from build123d import *

# Parameters (mm, degrees)
AUFSATZ_LINEAR_AUSTRAGEN1_DEPTH      = 10
SCHNITT_LINEAR_START                 = -0.7
SCHNITT_LINEAR_AUSTRAGEN1_DEPTH      = 0.7
SKIZZE5_W                            = 196
SKIZZE5_H                            = 8.65
AUFSATZ_LINEAR_AUSTRAGEN2_DEPTH      = 10
SCHNITT_LINEAR_AUSTRAGEN2_DEPTH      = 0.7
SCHNITT_LINEAR_AUSTRAGEN3_DEPTH      = 10
SCHNITT_LINEAR_AUSTRAGEN3_DEPTH_BACK = 10
BOHRUNG1_D                           = 6
BOHRUNG2_D                           = 4.134
BOHRUNG2_DEPTH                       = 10
BOHRUNG2_CSINK_D                     = 5
BOHRUNG2_CSINK_ANGLE                 = 90
BOHRUNG3_D                           = 4.134
BOHRUNG3_DEPTH                       = 10
BOHRUNG3_CSINK_D                     = 5
BOHRUNG3_CSINK_ANGLE                 = 90


with BuildPart() as part:
    # Skizze1 → Rotation1 (revolve)
    with BuildSketch(Plane.XY, mode=Mode.PRIVATE) as rotation1_sk:
        with BuildLine():
            Line((0, 0), (0, 6.8))
            Line((0, 6.8), (0.2, 7))
            Line((0.2, 7), (1, 7))
            Line((1, 7), (2, 8))
            Line((2, 8), (11.95, 8))
            Line((11.95, 8), (12.865685425, 7.084314575))
            ThreePointArc((12.865685425, 7.084314575), (13.125224104, 6.910896374), (13.43137085, 6.85))
            Line((13.43137085, 6.85), (14.2, 6.85))
            ThreePointArc((14.2, 6.85), (14.765685425, 7.084314575), (15, 7.65))
            Line((15, 7.65), (15, 8))
            Line((15, 8), (17, 8))
            Line((17, 8), (17, 0))
            Line((17, 0), (0, 0))
        make_face()
    revolve(rotation1_sk.sketch.rotate(Axis((17, 0, 0), (-1, 0, 0)), 270), axis=Axis((17, 0, 0), (-1, 0, 0)))

    # Skizze2 → Aufsatz-Linear austragen1 (add)
    with BuildSketch(Plane(origin=(17, 0, 0), x_dir=(0, 0, -1), z_dir=(1, 0, 0))):
        with BuildLine():
            Line((4.75, 8.977054082), (4.75, 9.6))
            ThreePointArc((4.75, 9.6), (4.632842712, 9.882842712), (4.35, 10))
            Line((4.35, 10), (-4.35, 10))
            ThreePointArc((-4.35, 10), (-4.632842712, 9.882842712), (-4.75, 9.6))
            Line((-4.75, 9.6), (-4.75, 8.977054082))
            ThreePointArc((-4.75, 8.977054082), (-4.791034545, 8.825604773), (-4.902912621, 8.715586488))
            ThreePointArc((-4.902912621, 8.715586488), (0, -10), (4.902912621, 8.715586488))
            ThreePointArc((4.902912621, 8.715586488), (4.791034545, 8.825604773), (4.75, 8.977054082))
        make_face()
    extrude(amount=AUFSATZ_LINEAR_AUSTRAGEN1_DEPTH)

    # Skizze3 → Schnitt-Rotation1 (revolve, cut)
    with BuildSketch(Plane(origin=(23, 0, 0), x_dir=(0, 0, -1), z_dir=(1, 0, 0)), mode=Mode.PRIVATE) as schnitt_rotation1_sk:
        Polygon((6.5, 9.5), (8.25, 9.5), (8.25, 5.4), (8, 5.4), (8, 5.3), (7.8, 5.5), (6.5, 5.5), align=None)
    revolve(schnitt_rotation1_sk.sketch.rotate(Axis((23, 5.5, -6.5), (0, 1, 0)), 180), axis=Axis((23, 5.5, -6.5), (0, 1, 0)), mode=Mode.SUBTRACT)

    # Skizze4 → Schnitt-Linear austragen1 (cut)
    with BuildSketch(Plane(origin=(0, 5.5, 0), x_dir=(1, 0, 0), z_dir=(0, 1, 0)).offset(SCHNITT_LINEAR_START)):
        with BuildLine():
            Line((23.3, 5.030306154), (23.3, 7.969693846))
            ThreePointArc((23.3, 7.969693846), (23, 8), (22.7, 7.969693846))
            Line((22.7, 7.969693846), (22.7, 5.030306154))
            ThreePointArc((22.7, 5.030306154), (23, 5), (23.3, 5.030306154))
        make_face()
    extrude(amount=SCHNITT_LINEAR_AUSTRAGEN1_DEPTH, mode=Mode.SUBTRACT)

    # Skizze5 → Rotation2 (revolve)
    with BuildSketch(Plane.XY, mode=Mode.PRIVATE) as rotation2_sk:
        with Locations((125, 4.325)):
            Rectangle(SKIZZE5_W, SKIZZE5_H)
    revolve(rotation2_sk.sketch.rotate(Axis((223, 0, 0), (-1, 0, 0)), 270), axis=Axis((223, 0, 0), (-1, 0, 0)))

    # Skizze6 → Aufsatz-Linear austragen2 (add)
    with BuildSketch(Plane(origin=(223, 0, 0), x_dir=(0, 0, -1), z_dir=(1, 0, 0))):
        with BuildLine():
            Line((4.75, 8.977054082), (4.75, 9.6))
            ThreePointArc((4.75, 9.6), (4.632842712, 9.882842712), (4.35, 10))
            Line((4.35, 10), (-4.35, 10))
            ThreePointArc((-4.35, 10), (-4.632842712, 9.882842712), (-4.75, 9.6))
            Line((-4.75, 9.6), (-4.75, 8.977054082))
            ThreePointArc((-4.75, 8.977054082), (-4.791034545, 8.825604773), (-4.902912621, 8.715586488))
            ThreePointArc((-4.902912621, 8.715586488), (0, -10), (4.902912621, 8.715586488))
            ThreePointArc((4.902912621, 8.715586488), (4.791034545, 8.825604773), (4.75, 8.977054082))
        make_face()
    extrude(amount=AUFSATZ_LINEAR_AUSTRAGEN2_DEPTH)

    # Skizze7 → Schnitt-Rotation2 (revolve, cut)
    with BuildSketch(Plane(origin=(225.35, 0, 0), x_dir=(0, 0, -1), z_dir=(1, 0, 0)), mode=Mode.PRIVATE) as schnitt_rotation2_sk:
        Polygon((6.5, 9.5), (8.25, 9.5), (8.25, 5.4), (8, 5.4), (8, 5.3), (7.8, 5.5), (6.5, 5.5), align=None)
    revolve(schnitt_rotation2_sk.sketch.rotate(Axis((225.35, 5.5, -6.5), (0, 1, 0)), 180), axis=Axis((225.35, 5.5, -6.5), (0, 1, 0)), mode=Mode.SUBTRACT)

    # Skizze8 → Schnitt-Linear austragen2 (cut)
    with BuildSketch(Plane(origin=(0, 5.5, 0), x_dir=(1, 0, 0), z_dir=(0, 1, 0)).offset(SCHNITT_LINEAR_START)):
        with BuildLine():
            Line((225.65, 5.030306154), (225.65, 7.969693846))
            ThreePointArc((225.65, 7.969693846), (225.35, 8), (225.05, 7.969693846))
            Line((225.05, 7.969693846), (225.05, 5.030306154))
            ThreePointArc((225.05, 5.030306154), (225.35, 5), (225.65, 5.030306154))
        make_face()
    extrude(amount=SCHNITT_LINEAR_AUSTRAGEN2_DEPTH, mode=Mode.SUBTRACT)

    # Skizze9 → Rotation3 (revolve)
    with BuildSketch(Plane.XY, mode=Mode.PRIVATE) as rotation3_sk:
        with BuildLine():
            Line((233, 0), (233, 8))
            Line((233, 8), (235, 8))
            Line((235, 8), (235, 7.65))
            ThreePointArc((235, 7.65), (235.234314575, 7.084314575), (235.8, 6.85))
            Line((235.8, 6.85), (236.56862915, 6.85))
            ThreePointArc((236.56862915, 6.85), (236.874775896, 6.910896374), (237.134314575, 7.084314575))
            Line((237.134314575, 7.084314575), (238.05, 8))
            Line((238.05, 8), (248, 8))
            Line((248, 8), (249, 7))
            Line((249, 7), (249.8, 7))
            Line((249.8, 7), (250, 6.8))
            Line((250, 6.8), (250, 0))
            Line((250, 0), (233, 0))
        make_face()
    revolve(rotation3_sk.sketch.rotate(Axis((250, 0, 0), (-1, 0, 0)), 270), axis=Axis((250, 0, 0), (-1, 0, 0)))

    # Skizze10 → Schnitt-Linear austragen3 (cut, two sides: drawn at the far end of the back side and taken through both)
    with BuildSketch(Plane(origin=(0, 0, 0), x_dir=(1, 0, 0), z_dir=(0, 1, 0)).offset(-SCHNITT_LINEAR_AUSTRAGEN3_DEPTH_BACK)):
        Polygon((228, 18), (228, 6), (250, 6), (250, -6), (228, -6), (228, -18), (262, -18), (262, 18), align=None)
    extrude(amount=SCHNITT_LINEAR_AUSTRAGEN3_DEPTH + SCHNITT_LINEAR_AUSTRAGEN3_DEPTH_BACK, mode=Mode.SUBTRACT)

    # Bohrung1 (through all)
    with Locations(Plane(origin=(0, 0, -6), x_dir=(-1, 0, 0), z_dir=(0, 0, -1))):
        with Locations((-237, 0)):
            Hole(BOHRUNG1_D / 2)

    # Bohrung2
    with Locations(Plane(origin=(0, 10, 0), x_dir=(1, 0, 0), z_dir=(0, 1, 0))):
        with Locations((23, 0)):
            CounterSinkHole(BOHRUNG2_D / 2, BOHRUNG2_CSINK_D / 2, depth=BOHRUNG2_DEPTH, counter_sink_angle=BOHRUNG2_CSINK_ANGLE)

    # Bohrung3
    with Locations(Plane(origin=(0, 10, 0), x_dir=(1, 0, 0), z_dir=(0, 1, 0))):
        with Locations((227, 0)):
            CounterSinkHole(BOHRUNG3_D / 2, BOHRUNG3_CSINK_D / 2, depth=BOHRUNG3_DEPTH, counter_sink_angle=BOHRUNG3_CSINK_ANGLE)

    # Skizze17 → Schnitt-Rotation3 (revolve, cut)
    with BuildSketch(Plane.XY, mode=Mode.PRIVATE) as schnitt_rotation3_sk:
        Polygon((-5, 0), (-5, 3), (41.2, 3), (41.2, 8), (205.2, 8), (205.2, 0), align=None)
    revolve(schnitt_rotation3_sk.sketch.rotate(Axis((205.2, 0, 0), (-1, 0, 0)), 270), axis=Axis((205.2, 0, 0), (-1, 0, 0)), mode=Mode.SUBTRACT)


solid = part.part
Read the model definition and answer for the solid it produces. Units are mm, in the model's axes. A direction names the side the tool comes from. Coordinates: 2 decimals unless noted, no trailing zeros. Order: outer loops, then holes, each group sorted by start corner. A loop starts at its lowest first (then second) coordinate and runs counter-clockwise, first axis right, second up. Notation, with made-up numbers: M 84.25,13.25 L 113.25,13.25 A18 cw 113.25,42.25 Z; hole C 75,22 d3. An arc over 180 degrees is marked long. Put each result on its own line as item: value. Start each with the question number.
Item 1: Given pin 1 Ø10 at (x, y) = (199, -0.5) entering from -Z; pin 2 Ø0.5 at (x, z) = (24, -6.5) entering from +Y; pin 3 Ø1.5 at (x, z) = (191, 5.5) entering from +Y; pin 4 Ø3.5 at (x, z) = (228, 0.5) entering from +Y, each flat-ended and moving along its own axis, determine where each tip first touches the part or whether it passes through.
Item 2: Section A-A, the plane x = 107 is taken. Determine the outline of the cut face in (y, z), plus the area to 3 significant figures.
Item 3: For faces 4 (the face through (16.01, -7.81, -1.73)), 5 (the face through (227, 0, 0)), 6 (the face through (237.29, -7.24, -0.1)), 7 (the face through (243, -8, 0)), determine the directions among +Z, -Z, +X, -X, +Y, -Y from which every point of the face is accessible in a straight line to the end or side of a thin tool.
Item 4: Consider probe 1 along X at (y, z) = (7.05, -6.5); probe 2 along Y at (x, z) = (124.5, 0); probe 3 along X at (y, z) = (8.75, 3.75). Determine where each line is inside the solid, lowest interval first. Write a range as [from, to].
Item 5: The mould has two halves that part along X. Classify faces 1 (the face through (239, 3, -6)), 2 (the face through (13.821, 2.058, 6.534)), 3 (the face through (248.8, 7.2, 0.1)): +X half, -X half, draft (parallel to the pull), parting line (faces both ways), or undercut.
Computed:
1. pin 1: stops at z = -8.65
1. pin 2: stops at y = 5.5
1. pin 3: stops at y = 7.23
1. pin 4: stops at y = 10
2. outline: C 0,0 d17.3; hole C 0,0 d16
2. area: 34.0 mm2
3. face 4: -X
3. face 5: +Y
3. face 6: -Y
3. face 7: +X, -Y
4. probe 1: x = [17, 21.25], [24.75, 27], [223, 223.6], [227.1, 228]
4. probe 2: y = [-8.65, -8], [8, 8.65]
4. probe 3: x = [17, 27], [223, 233]
5. face 1: draft
5. face 2: undercut
5. face 3: +X half
